Here's the drawing with two shaded views (mm, measured from the low corner). I have some questions. A direction names the side the tool comes from. Coordinates: 2 decimals unless noted, no trailing zeros. Loops run counter-clockwise (first coordinate to the right, second up) from the corner with the lowest first, then second, coordinate; pieces in that order, holes last. Notation, with made-up numbers: (-27, 7.25) - (6, 7.25) arc R11 cw to (6, 22.25) - close; hole circle Ø7 at (-7.5, 29). An arc over 180 degrees is marked (long way). Use a Markdown table: item, result.
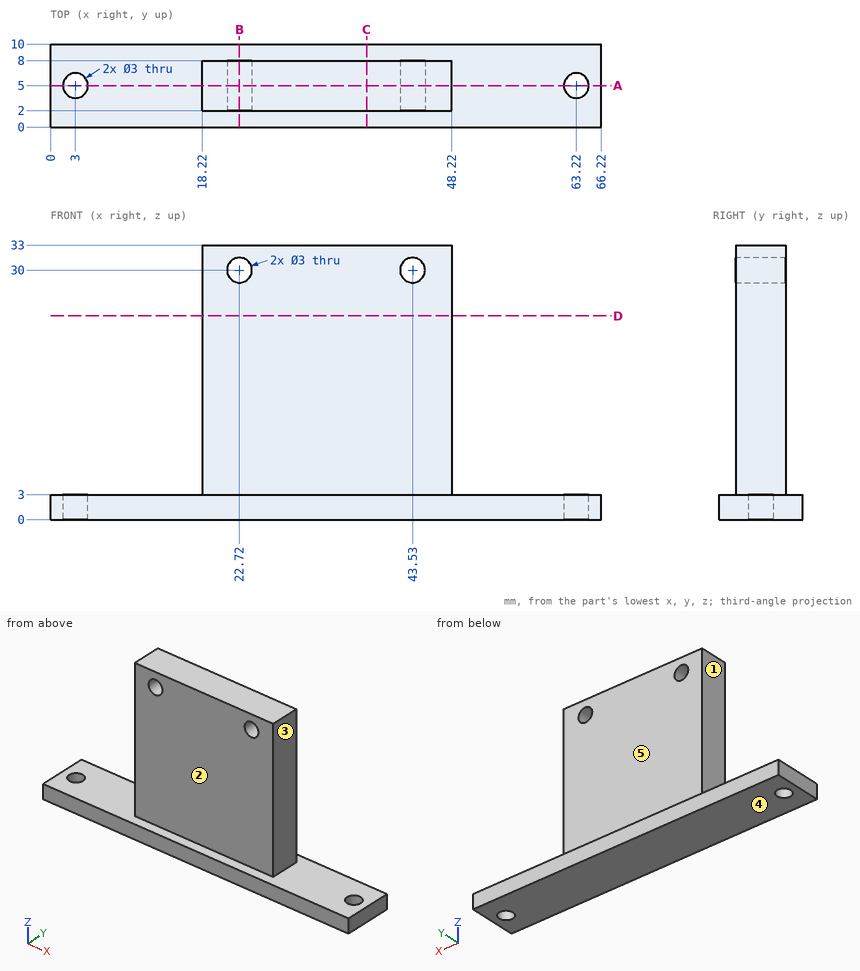
Q1. I want a section at D-D, the plane z = 24.5. Write out the boundary of the cut face in (x, y), then the cut area to 3 significant figures.
Check values:
| item | result |
|---|---|
| outline | (18.22, 2) - (48.22, 2) - (48.22, 8) - (18.22, 8) - close |
| area | 180 mm^2 |
Q2. I want a section at B-B, the plane x = 22.72. Write out the boundary of the cut face in (y, z).
Check values:
| item | result |
|---|---|
| outline | (0, 0) - (10, 0) - (10, 3) - (8, 3) - (8, 28.5) - (2, 28.5) - (2, 3) - (0, 3) - close; (2, 31.5) - (8, 31.5) - (8, 33) - (2, 33) - close |
Q3. I want a section at A-A, the plane y = 5. Write out the boundary of the cut face in (x, z), then the cut area to 3 significant figures.
Check values:
| item | result |
|---|---|
| outline | (0, 0) - (1.5, 0) - (1.5, 3) - (0, 3) - close; (4.5, 0) - (61.72, 0) - (61.72, 3) - (48.22, 3) - (48.22, 33) - (18.22, 33) - (18.22, 3) - (4.5, 3) - close; (64.72, 0) - (66.22, 0) - (66.22, 3) - (64.72, 3) - close; hole circle Ø3 at (22.72, 30); hole circle Ø3 at (43.53, 30) |
| area | 1,070 mm^2 |
Q4. Which directions (+Z, -Z, +X, -X, +Y, -Y) give clear straight access to the entire face, cutting with the end or side of a thin tool? Please do the marked faces 1, 2, 3, 4 and 5.
Check values:
| item | result |
|---|---|
| face 1 | +Z, -X, +Y, -Y |
| face 2 | +Z, +X, -X, -Y |
| face 3 | +Z, +X, +Y, -Y |
| face 4 | -Z, +X, -X, +Y, -Y |
| face 5 | +Z, +X, -X, +Y |
Q5. Please list where these lines run through material, in increasing order: L1, parallel to X at y = 5.8, z = 30; L2, parallel to X at y = 2.5, z = 31; L3, parallel to Y at x = 63.22, z = 1.85. Write a range as from..to.
Check values:
| item | result |
|---|---|
| L1 | 18.22..21.22, 24.22..42.03, 45.03..48.22 |
| L2 | 18.22..21.6, 23.84..42.41, 44.65..48.22 |
| L3 | 0..3.5, 6.5..10 |
Q6. I want a section at C-C, the plane x = 38. Write out the boundary of the cut face in (y, z).
Check values:
| item | result |
|---|---|
| outline | (0, 0) - (10, 0) - (10, 3) - (8, 3) - (8, 33) - (2, 33) - (2, 3) - (0, 3) - close |
Q7. Will these pins go through, and if not, where does the flat tip stop? P1, Ø3, axis at x = 36, z = 16, coming from the +Y side; P2, Ø1.5, axis at x = 56.5, y = 6.5, coming from the +Z side; P3, Ø15, axis at x = 28, z = 21.5, coming from the -Y side; P4, Ø2.5, axis at x = 63.22, y = 5, coming from the -Z side.
Check values:
| item | result |
|---|---|
| P1 | y = 8 |
| P2 | z = 3 |
| P3 | y = 2 |
| P4 | through |
